Autodesk Inventor part; units mm, degrees
ref_plane "YZ Plane" through (0, 0, 0) normal (1, 0, 0) x (0, 1, 0)
ref_plane "XZ Plane" through (0, 0, 0) normal (0, 1, 0) x (-1, 0, 0)
ref_plane "XY Plane" through (0, 0, 0) normal (0, 0, 1) x (1, 0, 0)
sketch "Sketch1" plane through (0, 0, 0) normal (0, 0, 1) x (1, 0, 0)
  circle A0 centre (0, 0) radius 2.75
  circle A1 centre (-22, 22) radius 2.75
  circle A2 centre (0, 0) radius 11 construction
  circle A3 centre (-22, 22) radius 11 construction
  line L0 (-41.3602, 39.2963) -> (24.6813, 39.2963)
  line L1 (24.6813, 39.2963) -> (24.6813, -18.4462)
  line L2 (24.6813, -18.4462) -> (-41.3602, -18.4462)
  line L3 (-41.3602, -18.4462) -> (-41.3602, 39.2963)
  dimension "d0" = 5.5
  dimension "d1" = 5.5
  dimension "d2" = 22
  dimension "d3" = 22
  dimension "d4" = 22
extrude "Extrusion1" add sketch "Sketch1" against normal blind 10
properties part number "rearSwingarmBaseV1"
Here's how the part is built. I have some questions about the finished solid (model axes, mm). Give positions to 0.01 mm unless a question says otherwise; leave off trailing zeros. Write each loop counter-clockwise with the first axis right and the second up, starting at its lowest first coordinate (ties: lowest second). Pieces come first, ordered by that corner, then holes. Notation, with made-up numbers: (38.5, -29) -> (93.5, -29) arc R27 ccw to (93.5, -10) -> close; hole circle Ø11 at (5.25, 82). An arc over 180 degrees is marked (long way). Use one line per item in the form item = value. Start each with the question number.
1. Thinking about a two-plate mould opening in X: for faces 1 (the face through (-41.36, 10, -5)), 2 (the face through (-24.747, 22.121, -4.93)), 3 (the face through (-9, 11, -10)), 4 (the face through (24.681, 11, -5)), which applies, +X half, -X half, draft (parallel to the pull), parting line (faces both ways), or undercut?
2. Imagine slicing it at A-A on x = -22. List the corners of the cut face in (y, z) for me.
3. If I drill on L1, parallel to Y at x = -22, z = -6; L2, parallel to Y at x = 0, z = -4.75; L3, parallel to X at y = -2, z = -8.5, over which ranges is the centre line in solid material (lowest first)?
4. Imagine slicing it at B-B on y = 22. List the corners of the cut face in (x, z) for me.
5. Will these pins go through, and if not, where does the flat tip stop? pin 1 Ø2 at (x, y) = (-22.5, 5.5) entering from +Z; pin 2 Ø3.5 at (x, y) = (0, 0) entering from +Z.
Entries:
q1.face_1 = -X half
q1.face_2 = undercut
q1.face_3 = draft
q1.face_4 = +X half
q2.outline = (-18.45, -10) -> (19.25, -10) -> (19.25, 0) -> (-18.45, 0) -> close; (24.75, -10) -> (39.3, -10) -> (39.3, 0) -> (24.75, 0) -> close
q3.L1 = -18.45 to 19.25, 24.75 to 39.3
q3.L2 = -18.45 to -2.75, 2.75 to 39.3
q3.L3 = -41.36 to -1.89, 1.89 to 24.68
q4.outline = (-41.36, -10) -> (-24.75, -10) -> (-24.75, 0) -> (-41.36, 0) -> close; (-19.25, -10) -> (24.68, -10) -> (24.68, 0) -> (-19.25, 0) -> close
q5.pin_1 = 0
q5.pin_2 = through
